Verification items for the finished model (mm, model axes). A direction names the side the tool comes from. Round coordinates to 2 decimals unless told otherwise and drop trailing zeros. Write each loop counter-clockwise with the first axis right and the second up, starting at its lowest first coordinate (ties: lowest second). Pieces come first, ordered by that corner, then holes. Notation, with made-up numbers: (47, 21.25) - (59, 21.25) arc R17 ccw to (59, 25.25) - close; hole circle Ø10 at (-9.5, -34.75). An arc over 180 degrees is marked (long way). Answer as a JSON object with one key per item and string values.
```python
from build123d import *

# Parameters (mm, degrees)
SKETCH1_R           = 6.5
BOSS_EXTRUDE1_DEPTH = 8.5
BOSS_EXTRUDE1_TAPER = 15
SKETCH2_R           = 5.1
CUT_EXTRUDE1_DEPTH  = 2.25
FILLET1_R           = 2


# Read off the part's stored shape, not the designer's step: Shell2
with BuildPart() as part:
    # Sketch1 → Boss-Extrude1 (new body)
    with BuildSketch(Plane(origin=(0, 0, 0), x_dir=(1, 0, 0), z_dir=(0, 1, 0))):
        Circle(SKETCH1_R)
    extrude(amount=BOSS_EXTRUDE1_DEPTH, taper=BOSS_EXTRUDE1_TAPER)

    # Sketch2 → Cut-Extrude1 (cut)
    with BuildSketch(Plane.XZ):
        with Locations(Location((0, 0, 0), (0, 0, 270))):
            Circle(SKETCH2_R)
    extrude(amount=-CUT_EXTRUDE1_DEPTH, mode=Mode.SUBTRACT)

    # Fillet1
    fillet1_edges = [part.edges().sort_by_distance(p)[0] for p in [
        (-4.222431864, 8.5, 0),
    ]]
    fillet(fillet1_edges, radius=FILLET1_R)

    # Shell2 outline → Shell2 (revolve, cut)
    with BuildSketch(Plane.XY):
        with BuildLine():
            Line((4.70654671, 2.25), (3.508814841, 6.719996188))
            ThreePointArc((3.508814841, 6.719996188), (3.205225103, 7.174350339), (2.687777888, 7.35))
            Line((2.687777888, 7.35), (0, 7.35))
            Line((0, 7.35), (0, 2.25))
            Line((0, 2.25), (4.70654671, 2.25))
        make_face()
    revolve(axis=Axis((0, 0, 0), (0, 1, 0)), mode=Mode.SUBTRACT)


solid = part.part
```
Q1. Gauge pin test, flat ends, axial feed: P1, Ø4, axis at x = 4, y = 7, coming from the +Z side; P2, Ø1, axis at x = -2, y = 6.5, coming from the +Z side; P3, Ø2, axis at x = 2.5, y = 4.5, coming from the -Z side. Record the tip position at first contact, or that the pin passes through.
Geometry check:
{"P1": "stops at z = 4.33", "P2": "stops at z = 4.57", "P3": "stops at z = -5.18"}
Q2. Section check C-C, the plane y = 4. Record the cut outline in (x, z), then the cut area to 3 significant figures.
Geometry check:
{"outline": "circle Ø10.86 at (0, 0); hole circle Ø8.48 at (0, 0)", "area": "36.2 mm2"}
Q3. Section check A-A, the plane x = 0. Record the cut outline in (y, z), then the cut area to 3 significant figures.
Geometry check:
{"outline": "(0, -6.5) - (7.02, -4.62) arc R2 ccw to (8.5, -2.69) - (8.5, 2.69) arc R2 ccw to (7.02, 4.62) - (0, 6.5) - (0, 5.1) - (2.25, 5.1) - (2.25, 4.71) - (6.72, 3.51) arc R0.85 cw to (7.35, 2.69) - (7.35, -2.69) arc R0.85 cw to (6.72, -3.51) - (2.25, -4.71) - (2.25, -5.1) - (0, -5.1) - close", "area": "26.4 mm2"}
Q4. Section check B-B, the plane y = 0.75. Record the cut outline in (x, z).
Geometry check:
{"outline": "circle Ø12.6 at (0, 0); hole circle Ø10.2 at (0, 0)"}
Q5. Set-up check for faces 4 (the cylindrical face through (1.532, 1.109, -4.864)), 5 (the flat face through (0, 8.5, 0)): record each of +Z, -Z, +X, -X, +Y, -Y from which the full face is reachable in a straight line by a thin tool's end or side.
Geometry check:
{"face 4": "-Y", "face 5": "+Z, -Z, +X, -X, +Y"}
Q6. Release check for a two-part mould opening along Z. For faces 1 (the conical face through (-4.07, 5.12, 3.12)), 2 (the flat face through (-4.4, 0, 2.9)), 3 (the flat face through (0, 7.35, 0)) record: released by +Z, released by -Z, zero draft, split by the parting line, or undercut.
Geometry check:
{"face 1": "split by the parting line", "face 2": "zero draft", "face 3": "undercut"}
Q7. Material ranges on line 1 along Z through (x, y) = (-0.75, 5.5); line 2 along Z through (x, y) = (2.75, 5); line 3 along X through (y, z) = (6, 3), recorded low to high. Write a range as [from, to].
Geometry check:
{"line 1": "z = [-4.97, -3.76], [3.76, 4.97]", "line 2": "z = [-4.37, -2.86], [2.86, 4.37]", "line 3": "x = [-3.86, -2.17], [2.17, 3.86]"}
